Autodesk Inventor part; units mm, degrees
ref_plane "Work Plane2" through (-40.9959, 0.8639, 22.2359) normal (0, 0, 1) x (1, 0, 0)
ref_plane "YZ Plane" through (0, 0, 0) normal (1, 0, 0) x (0, 1, 0)
ref_plane "XZ Plane" through (0, 0, 0) normal (0, 1, 0) x (-1, 0, 0)
ref_plane "Work Plane1" through (0, 0, 10) normal (0, 0, 1) x (1, 0, 0)
sketch "Sketch1" plane through (0, 0, 10) normal (0, 0, 1) x (1, 0, 0)
  line L0 (-4.0299, -0.3538) -> (-2.2322, 1.4439) construction
  arc A0 (-1.4439, 2.2322) -> (-2.2322, 1.4439) centre (-0.9299, 0.9299) ccw construction
  line L1 (-1.4439, 2.2322) -> (0.3538, 4.0299) construction
  line L2 (-37.8299, 42.8299) -> (-37.8299, 37.8299) construction
  line L3 (-37.8299, 37.8299) -> (-42.9208, 37.8299) construction
  line L4 (-37.8299, 42.2137) -> (-37.8299, 45.8299) construction
  line L5 (-37.8299, 45.8299) -> (-4.0299, 45.8299) construction
  line L6 (-4.0299, 45.8299) -> (-4.0299, 42.2137) construction
  line L7 (-4.0299, 4.0299) -> (0.3538, 4.0299)
  circle A1 centre (-20.9299, 20.9299) radius 17.5
  line L8 (-20.9299, 58.9723) -> (17.1124, 20.9299) construction
  line L9 (17.1124, 20.9299) -> (-20.9299, -17.1124) construction
  line L10 (-20.9299, -17.1124) -> (-58.9723, 20.9299) construction
  line L11 (-58.9723, 20.9299) -> (-20.9299, 58.9723) construction
  line L12 (-20.9299, 58.9723) -> (-20.9299, -17.1124) construction
  line L13 (17.1124, 20.9299) -> (-58.9723, 20.9299) construction
  line L14 (-20.9299, 58.9723) -> (32.8701, 58.9723) construction
  line L15 (-43.4299, 43.4299) -> (1.5701, 43.4299) construction
  line L16 (1.5701, 43.4299) -> (1.5701, -1.5701) construction
  line L17 (1.5701, -1.5701) -> (-43.4299, -1.5701) construction
  line L18 (-43.4299, -1.5701) -> (-43.4299, 43.4299) construction
  line L19 (-43.4299, 43.4299) -> (1.5701, -1.5701) construction
  line L20 (1.5701, 43.4299) -> (-43.4299, -1.5701) construction
  line L21 (-43.4299, 5.3876) -> (-43.4299, 36.4723)
  line L22 (-43.4299, 36.4723) -> (-36.4723, 43.4299)
  line L23 (-36.4723, 43.4299) -> (-5.3876, 43.4299)
  line L24 (-5.3876, 43.4299) -> (1.5701, 36.4723)
  line L25 (1.5701, 36.4723) -> (1.5701, 5.3876)
  line L26 (1.5701, 5.3876) -> (-5.3876, -1.5701)
  line L27 (-5.3876, -1.5701) -> (-36.4723, -1.5701)
  line L28 (-36.4723, -1.5701) -> (-43.4299, 5.3876)
  line L29 (-4.0299, 42.2137) -> (-37.8299, 42.2137)
  line L30 (-4.0299, -0.3538) -> (-4.0299, 4.0299)
  point P0 (-37.8299, 4.0299)
  point P1 (-20.9299, 20.9299)
  dimension "d18" = 53.8
  dimension "d19" = 45
  dimension "d20" = 53.8
  dimension "d21" = 45
  dimension "d22" = 45
extrude "Extrusion1" add sketch "Sketch1" along normal blind 3
sketch "Sketch2" plane through (0, 0, 13) normal (0, 0, 1) x (1, 0, 0)
  circle A0 centre (-35.9299, 35.9299) radius 3.0099 construction
  circle A1 centre (-5.93, 35.9299) radius 3.0099 construction
  circle A2 centre (-5.93, 5.93) radius 3.0099 construction
  circle A3 centre (-35.9299, 5.93) radius 3.0099 construction
  circle A4 centre (-35.9299, 35.9299) radius 2.7099
  circle A5 centre (-5.93, 35.9299) radius 2.7099
  circle A6 centre (-5.93, 5.93) radius 2.7099
  circle A7 centre (-35.9299, 5.93) radius 2.7099
  circle A8 centre (-20.9299, 20.9299) radius 17.5
  line L0 (-20.9299, 42.1431) -> (0.2833, 20.9299)
  line L1 (0.2833, 20.9299) -> (-20.9299, -0.2833)
  line L2 (-20.9299, -0.2833) -> (-42.1431, 20.9299)
  line L3 (-42.1431, 20.9299) -> (-20.9299, 42.1431)
  line L4 (-20.9299, 42.1431) -> (-20.9299, -0.2833) construction
  line L5 (0.2833, 20.9299) -> (-42.1431, 20.9299) construction
  line L6 (-20.9299, 42.1431) -> (9.0701, 42.1431) construction
  circle A9 centre (-20.9299, 42.1431) radius 2.71
  circle A10 centre (0.2833, 20.9299) radius 2.71
  circle A11 centre (-20.9299, -0.2833) radius 2.71
  circle A12 centre (-42.1431, 20.9299) radius 2.71
  point P0 (0, 0)
  dimension "d_1" = 0.3
  dimension "d13" = 0.3
  dimension "d14" = 0.3
  dimension "d15" = 0.3
  dimension "d30" = 30
  dimension "d31" = 45
  dimension "d32" = 30
  dimension "a1" = 5.42
  dimension "d34" = 5.42
  dimension "d35" = 5.42
  dimension "d36" = 5.42
ref_plane "Work Plane2" through (-40.9959, 0.8639, 22.2359) normal (0, 0, 1) x (1, 0, 0)
extrude "Extrusion2" add sketch "Sketch2" along normal up to surface (9.2359 mm away) contours A10 L1 L0 | L0 L1 A10 | A9 L3 L0 | L0 L3 A9 | A11 L2 L1 | L1 L2 A11 | A12 L2 L3 | L3 L2 A12
sketch "Sketch3" plane through (0, 0, 10) normal (0, 0, -1) x (-1, 0, 0)
  line L0 (37.8299, -0.4701) -> (37.8299, 4.0299) construction
  line L1 (4.0299, 4.0299) -> (4.0299, -0.4701) construction
  line L2 (37.8299, -0.4701) -> (37.8299, 1.1886) construction
  line L3 (4.0299, -3.9701) -> (4.0299, -0.3538) construction
  line L4 (45.8299, 4.0299) -> (42.2137, 4.0299) construction
  line L5 (-0.3538, 4.0299) -> (-3.9701, 4.0299) construction
  line L6 (-3.9701, 37.8299) -> (-0.3538, 37.8299) construction
  line L7 (4.0299, 42.2137) -> (4.0299, 45.8299) construction
  line L8 (37.8299, 45.8299) -> (37.8299, 42.2137) construction
  line L9 (42.2137, 37.8299) -> (45.8299, 37.8299) construction
  line L10 (37.8299, 37.7299) -> (45.8299, 37.7299)
  line L11 (45.8299, 37.7299) -> (45.8299, 4.1299)
  line L12 (45.8299, 4.1299) -> (37.8299, 4.1299)
  line L13 (37.8299, 4.1299) -> (37.8299, 37.7299)
  line L14 (37.7299, 4.0299) -> (4.1299, 4.0299)
  line L15 (4.1299, 4.0299) -> (4.1299, -3.9701)
  line L16 (4.1299, -3.9701) -> (37.7299, -3.9701)
  line L17 (37.7299, -3.9701) -> (37.7299, 4.0299)
  line L18 (4.0299, 4.1299) -> (-3.9701, 4.1299)
  line L19 (-3.9701, 4.1299) -> (-3.9701, 37.7299)
  line L20 (-3.9701, 37.7299) -> (4.0299, 37.7299)
  line L21 (4.0299, 37.7299) -> (4.0299, 4.1299)
  line L22 (4.1299, 37.8299) -> (37.7299, 37.8299)
  line L23 (37.7299, 37.8299) -> (37.7299, 45.8299)
  line L24 (37.7299, 45.8299) -> (4.1299, 45.8299)
  line L25 (4.1299, 45.8299) -> (4.1299, 37.8299)
  point P0 (0, 0)
  dimension "d23" = 0.1
  dimension "d24" = 0.1
  dimension "d25" = 0.1
  dimension "d26" = 0.1
  dimension "d27" = 0.1
extrude "Extrusion3" add sketch "Sketch3" against normal up to surface (3 mm away)
equation "\"d13\" = d_1"
equation "\"d14\" = d_1"
equation "\"d15\" = d_1"
equation "\"d34\" = a1"
equation "\"d35\" = a1"
equation "\"d36\" = a1"
properties part number "50_Cube_Insert_Thorlabs"
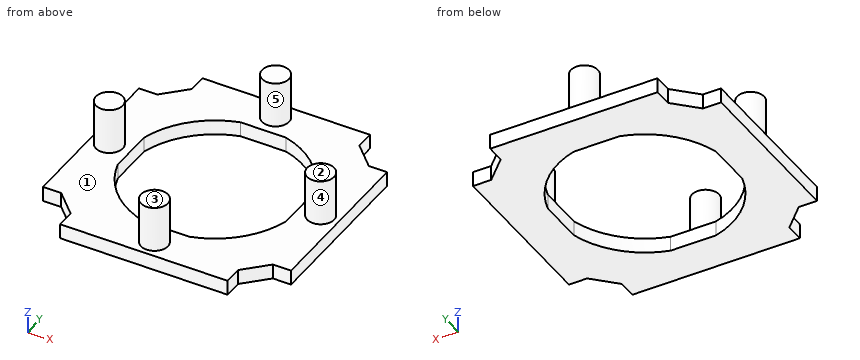
Part model, mm, in its own coordinate system. Face numbers are marked on the shaded views. A direction names the side the tool comes from. Coordinates: 2 decimals unless noted, no trailing zeros. Loops run counter-clockwise (first coordinate to the right, second up) from the corner with the lowest first, then second, coordinate; pieces in that order, holes last. Notation, with made-up numbers: (81, -2) -> (100, -2) arc R27 ccw to (100, 24) -> close; hole circle Ø7 at (42.5, 18.5). An arc over 180 degrees is marked (long way). Use a Markdown table: item, result. Add a question column.
Item 1: Band-saw the part on B-B on x = -36. Write the cut outline in (y, z), plus the area to 3 significant figures.
Item 2: Band-saw the part on D-D on x = -1. Write the cut outline in (y, z), plus the area to 3 significant figures.
Item 3: Probe probe 1 along X at (y, z) = (17, 11.75); probe 2 along Z at (x, y) = (-3.5, 36.5); probe 3 along X at (y, z) = (9, 12). List the from-to ranges inside material, lowest first.
Item 4: Flat gauge pins, fed straight in: P1, Ø8, axis at x = -2, y = 3.5, coming from the +Z side; P2, Ø4, axis at y = 1.5, z = 11.5, coming from the +X side; P3, Ø3, axis at x = -3, z = 18.5, coming from the +Y side. Where does each tip first touch, or does it go through?
Item 5: Band-saw the part on C-C on z = 18.5. Write the cut outline in (x, y).
Item 6: Which spindle directions (+Z, -Z, +X, -X, +Y, -Y) get a long thin tool onto all of the face, cutting with end or side? Do the marked faces 1 and 2. Say none if no direction does.
Item 7: Pull direction Y, two halves, no side cores. Call the marked faces 3, 4 and 5: +Y half, -Y half, draft (parallel to the pull), parting line (faces both ways), or undercut.
Item 8: Band-saw the part on A-A on y = 12. Write the cut outline in (x, z), plus the area to 3 significant figures.
Geometry says:
| question | item | result |
|---|---|---|
| 1 | outline | (-3.97, 10) -> (12.03, 10) -> (12.03, 13) -> (-3.97, 13) -> close; (29.83, 10) -> (45.83, 10) -> (45.83, 13) -> (29.83, 13) -> close |
| 1 | area | 96.0 mm² |
| 2 | outline | (2.82, 10) -> (39.04, 10) -> (39.04, 13) -> (23.32, 13) -> (23.32, 22.24) -> (18.54, 22.24) -> (18.54, 13) -> (2.82, 13) -> close |
| 2 | area | 153 mm² |
| 3 | probe 1 | -45.83 to -37.83, -4.03 to 3.97 |
| 3 | probe 2 | 10 to 13 |
| 3 | probe 3 | -45.83 to -33.73, -8.13 to 3.97 |
| 4 | P1 | z = 13 |
| 4 | P2 | x = -0.32 |
| 4 | P3 | y = 22.97 |
| 5 | outline | circle Ø5.42 at (-42.14, 20.93); circle Ø5.42 at (-20.93, -0.28); circle Ø5.42 at (-20.93, 42.14); circle Ø5.42 at (0.28, 20.93) |
| 6 | face 1 | +Z |
| 6 | face 2 | +Z, +X, -X, +Y, -Y |
| 7 | face 3 | draft |
| 7 | face 4 | parting line |
| 7 | face 5 | undercut |
| 8 | outline | (-45.83, 10) -> (-35.98, 10) -> (-35.98, 13) -> (-45.83, 13) -> close; (-5.88, 10) -> (3.97, 10) -> (3.97, 13) -> (-5.88, 13) -> close |
| 8 | area | 59.1 mm² |
